```python
from build123d import *

# Parameters (mm, degrees)
ESQUISSE1_R                  = 4.75
MAIN_EXTRUSION_DEPTH         = 5
GEAR_ELEMENT_DEPTH           = 5
R_P_TITION_CIRCULAIRE1_COUNT = 8
ESQUISSE3_R                  = 3
MAIN_AXE_DEPTH               = 15
ESQUISSE4_W                  = 4
ESQUISSE4_H                  = 1
AXE_TRAIT_DEPTH              = 3


with BuildPart() as part:
    # Esquisse1 → Main Extrusion (new body)
    with BuildSketch(Plane.XY):
        Circle(ESQUISSE1_R)
    extrude(amount=MAIN_EXTRUSION_DEPTH)

    # Esquisse2 → Gear Element (add)
    with BuildSketch(Plane.XY.offset(5)):
        Polygon((-1.25, 4.582575695), (1.25, 4.582575695), (0.75, 6.582575695), (-0.75, 6.582575695), align=None)
    gear_element = extrude(amount=-GEAR_ELEMENT_DEPTH)

    # Répétition circulaire1: Gear Element ×8 about axis
    r_p_tition_circulaire1_axis = Axis((0, 0, 0), (0, 0, 1))
    for i in range(1, R_P_TITION_CIRCULAIRE1_COUNT):
        add(gear_element.rotate(r_p_tition_circulaire1_axis, i * 360 / R_P_TITION_CIRCULAIRE1_COUNT))

    # Esquisse3 → Main Axe (add)
    with BuildSketch(Plane(origin=(0, 0, 0), x_dir=(-1, 0, 0), z_dir=(0, 0, -1))):
        Circle(ESQUISSE3_R)
    extrude(amount=MAIN_AXE_DEPTH)

    # Esquisse4 → Axe Trait (cut)
    with BuildSketch(Plane(origin=(0, 0, -15), x_dir=(-1, 0, 0), z_dir=(0, 0, -1))):
        Rectangle(ESQUISSE4_W, ESQUISSE4_H)
    extrude(amount=-AXE_TRAIT_DEPTH, mode=Mode.SUBTRACT)


solid = part.part
```
Geometry check sheet. Reference: the model listing, model coordinates, mm. A direction names the side the tool comes from. Give positions to 0.01 mm unless a question says otherwise; leave off trailing zeros. Order: outer loops, then holes, each group sorted by start corner. A loop starts at its lowest first (then second) coordinate and runs counter-clockwise, first axis right, second up. Notation, with made-up numbers: (-11, -12) - (-7, -12) arc R21 cw to (-7, 8) - close; hole circle Ø11 at (-17.75, 24.5). An arc over 180 degrees is marked (long way). Write item = value, one per line. Start each with the question number.
1) Access from +Z, -Z, +X, -X, +Y, -Y to the whole of each face (thin tool, end or side, straight path). Record for faces 1 (the flat face through (2, 0, -14)), 2 (the flat face through (1.004, 5.569, 2.535)), 3 (the flat face through (5.597, 0.996, 2.535)), 4 (the flat face through (-4.65, 4.66, 2.54)), 5 (the flat face through (-5.597, -0.996, 2.535)).
2) Scan lines: L1, parallel to Y at x = -5, z = 1.75; L2, parallel to Y at x = 0, z = -2; L3, parallel to Z at x = -3.25, y = -3.75. Record each from-to range of solid material in increasing order.
3) Section check A-A (x = 0). Enter the section's corners in (y, z), then the cut area to 3 significant figures.
4) Draft check along Y on faces 6 (the flat face through (4.66, -3.25, 2.54)), 7 (the flat face through (4.65, -4.66, 2.54)), 8 (the flat face through (-2, 3, 0)). Enter one of: released by +Y, released by -Y, zero draft, split by the parting line, or undercut.
5) Section check C-C (z = -10). Enter the section's corners in (x, y), then the cut area to 3 significant figures.
6) Gauge pin test, flat ends, axial feed: pin 1 Ø1.5 at (x, z) = (-1, -13.5) entering from +Y; pin 2 Ø3.5 at (x, z) = (0.5, -14) entering from -Y; pin 3 Ø3 at (x, z) = (4, 3) entering from +Y; pin 4 Ø1.5 at (x, z) = (-4, -3.5) entering from -Y. Record the tip position at first contact, or that the pin passes through.
7) Section check B-B (y = 0). Enter the section's corners in (x, z).
8) Section check D-D (y = 1.5). Enter the section's corners in (x, z), then the cut area to 3 significant figures.
Geometry check:
q1.face_1 = -Z
q1.face_2 = +Z, -Z, +Y
q1.face_3 = +Z, -Z, +X
q1.face_4 = +Z, -Z, -X, +Y
q1.face_5 = +Z, -Z, -X
q2.L1 = -4.31 to -3.82, -1.15 to 1.15, 3.82 to 4.31
q2.L2 = -3 to 3
q2.L3 = 0 to 5
q3.outline = (-6.58, 0) - (-3, 0) - (-3, -15) - (-0.5, -15) - (-0.5, -12) - (0.5, -12) - (0.5, -15) - (3, -15) - (3, 0) - (6.58, 0) - (6.58, 5) - (-6.58, 5) - close
q3.area = 153 mm2
q4.face_6 = undercut
q4.face_7 = released by -Y
q4.face_8 = zero draft
q5.outline = circle Ø6 at (0, 0)
q5.area = 28.3 mm2
q6.pin_1 = 2.99
q6.pin_2 = -3
q6.pin_3 = 5.18
q6.pin_4 = through
q7.outline = (-6.58, 0) - (-3, 0) - (-3, -15) - (-2, -15) - (-2, -12) - (2, -12) - (2, -15) - (3, -15) - (3, 0) - (6.58, 0) - (6.58, 5) - (-6.58, 5) - close
q8.outline = (-4.51, 0) - (-2.6, 0) - (-2.6, -15) - (2.6, -15) - (2.6, 0) - (4.51, 0) - (4.51, 5) - (-4.51, 5) - close
q8.area = 123 mm2
